Input: dimensioned drawing with shaded views. Units: mm. Origin: part minimum x, y, z. Coordinates: 2 decimals unless noted, no trailing zeros. Loops run counter-clockwise (first coordinate to the right, second up) from the corner with the lowest first, then second, coordinate; pieces in that order, holes last.
(1) Section B-B, the plane x = 20. Return loops of the section in (y, z), then the cut area to 3 significant figures.
(2) Section A-A, the plane z = 4.25. Return loops of the section in (x, y).
(3) Mould query, pull axis X, two halves, no side actions, for the marked faces 1, 2, 3 and 4. Classes: released by +X, released by -X, zero draft, split by the parting line, or undercut.
(4) Line query: L1, parallel to X at y = 8, z = 16; L2, parallel to Y at x = 34.5, z = 14; L3, parallel to Y at x = 5, z = 1.5. Output: solid intervals per line, ascending.
(5) Section C-C, the plane y = 10. Return loops of the section in (x, z).
(6) Section D-D, the plane y = 35.5. Return loops of the section in (x, z), then the cut area to 3 significant figures.
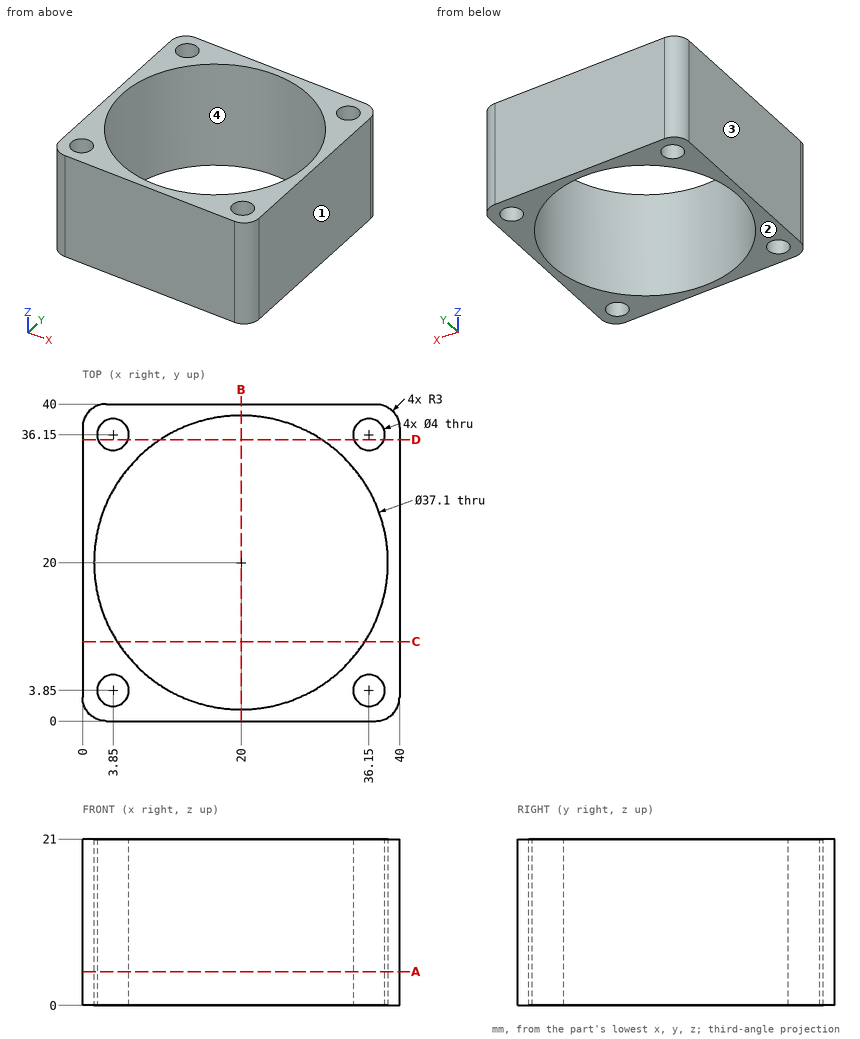
Report:
1. outline: (0, 0) - (1.45, 0) - (1.45, 21) - (0, 21) - close; (38.55, 0) - (40, 0) - (40, 21) - (38.55, 21) - close
1. area: 60.9 mm2
2. outline: (0, 3) arc R3 ccw to (3, 0) - (37, 0) arc R3 ccw to (40, 3) - (40, 37) arc R3 ccw to (37, 40) - (3, 40) arc R3 ccw to (0, 37) - close; hole circle Ø37.1 at (20, 20); hole circle Ø4 at (3.85, 3.85); hole circle Ø4 at (3.85, 36.15); hole circle Ø4 at (36.15, 3.85); hole circle Ø4 at (36.15, 36.15)
3. face 1: released by +X
3. face 2: zero draft
3. face 3: released by -X
3. face 4: undercut
4. L1: x = 0 to 5.85, 34.15 to 40
4. L2: y = 0 to 2.72, 4.98 to 8.43, 31.57 to 35.02, 37.28 to 40
4. L3: y = 0 to 2.21, 5.49 to 9.09, 30.91 to 34.51, 37.79 to 40
5. outline: (0, 0) - (4.38, 0) - (4.38, 21) - (0, 21) - close; (35.62, 0) - (40, 0) - (40, 21) - (35.62, 21) - close
6. outline: (0, 0) - (1.96, 0) - (1.96, 21) - (0, 21) - close; (5.74, 0) - (9.81, 0) - (9.81, 21) - (5.74, 21) - close; (30.19, 0) - (34.26, 0) - (34.26, 21) - (30.19, 21) - close; (38.04, 0) - (40, 0) - (40, 21) - (38.04, 21) - close
6. area: 253 mm2
